Here's how the part is built. I have some questions about the finished solid (model axes, mm). A direction names the side the tool comes from. Round coordinates to 2 decimals unless told otherwise and drop trailing zeros. Write each loop counter-clockwise with the first axis right and the second up, starting at its lowest first coordinate (ties: lowest second). Pieces come first, ordered by that corner, then holes. Notation, with made-up numbers: (48, -26.5) -> (67, -26.5) arc R20 ccw to (67, 2.5) -> close; hole circle Ø8 at (-31.5, 32.5). An arc over 180 degrees is marked (long way). Answer as CSV lines item,"result".
```python
from build123d import *

# Parameters (mm, degrees)
EXTRUDE_1_DEPTH   = 10
SKETCH_2_R        = 19
EXTRUDE_2_DEPTH   = 76
EXTRUDE_3_DEPTH   = 10
SKETCH_4_W        = 35
SKETCH_4_H        = 60
EXTRUDE_4_DEPTH   = 25
SKETCH_5_R        = 30
EXTRUDE_9_DEPTH   = 10
SKETCH_6_R        = 15
EXTRUDE_10_DEPTH  = 10
FILLET_1_R        = 5
SKETCH_7_R        = 7.5
EXTRUDE_11_DEPTH  = 8
SKETCH_8_W        = 30
SKETCH_8_H        = 30
EXTRUDE_12_DEPTH  = 37
FILLET_4_R        = 2
SKETCH_9_W        = 20
SKETCH_9_H        = 17.308382811
EXTRUDE_1_2_DEPTH = 20


with BuildPart() as part:
    # Sketch 1 → Extrude 1 (new body)
    with BuildSketch(Plane.XY):
        Polygon((-25.980762114, 0), (-12.990381057, -22.5), (12.990381057, -22.5), (25.980762114, 0), (12.990381057, 22.5), (-12.990381057, 22.5), align=None)
    extrude(amount=EXTRUDE_1_DEPTH)

    # Sketch 2 → Extrude 2 (add)
    with BuildSketch(Plane(origin=(0, 0, 0), x_dir=(-1, 0, 0), z_dir=(0, 0, -1))):
        with Locations(Location((0, 0, 0), (0, 0, 180))):
            Circle(SKETCH_2_R)
    extrude(amount=EXTRUDE_2_DEPTH)

    # Sketch 3 → Extrude 3 (add)
    with BuildSketch(Plane(origin=(0, 0, -76), x_dir=(-1, 0, 0), z_dir=(0, 0, -1))):
        Polygon((25.980762114, 0), (12.990381057, 22.5), (-12.990381057, 22.5), (-25.980762114, 0), (-12.990381057, -22.5), (12.990381057, -22.5), align=None)
    extrude(amount=EXTRUDE_3_DEPTH)

    # Sketch 4 → Extrude 4 (add)
    with BuildSketch(Plane(origin=(0, 0, 0), x_dir=(1, 0, 0), z_dir=(0, 1, 0))):
        with Locations((0, 38)):
            Rectangle(SKETCH_4_W, SKETCH_4_H)
    extrude(amount=EXTRUDE_4_DEPTH)

    # Sketch 5 → Extrude 9 (add)
    with BuildSketch(Plane(origin=(0, 25, 0), x_dir=(1, 0, 0), z_dir=(0, 1, 0))):
        with Locations(Location((0, 38, 0), (0, 0, 270))):
            Circle(SKETCH_5_R)
    extrude(amount=EXTRUDE_9_DEPTH)

    # Sketch 6 → Extrude 10 (add)
    with BuildSketch(Plane(origin=(0, 35, 0), x_dir=(1, 0, 0), z_dir=(0, 1, 0))):
        with Locations(Location((0, 38, 0), (0, 0, 270))):
            Circle(SKETCH_6_R)
    extrude(amount=EXTRUDE_10_DEPTH)

    # Fillet 1
    fillet_1_edges = [part.edges().sort_by_distance(p)[0] for p in [
        (0, 45, -53),
    ]]
    fillet(fillet_1_edges, radius=FILLET_1_R)

    # Sketch 7 → Extrude 11 (add)
    with BuildSketch(Plane(origin=(0, 45, 0), x_dir=(1, 0, 0), z_dir=(0, 1, 0))):
        with Locations(Location((0, 38, 0), (0, 0, 270))):
            Circle(SKETCH_7_R)
    extrude(amount=EXTRUDE_11_DEPTH)

    # Sketch 8 → Extrude 12 (add)
    with BuildSketch(Plane(origin=(0, 53, 0), x_dir=(1, 0, 0), z_dir=(0, 1, 0))):
        with Locations((0, 38)):
            Rectangle(SKETCH_8_W, SKETCH_8_H)
    extrude(amount=EXTRUDE_12_DEPTH)

    # Fillet 4
    fillet_4_edges = [part.edges().sort_by_distance(p)[0] for p in [
        (0, 35, -68),
    ]]
    fillet(fillet_4_edges, radius=FILLET_4_R)

    # Sketch 9 → Extrude 1 2 (add)
    with BuildSketch(Plane(origin=(0, 0, -53), x_dir=(-1, 0, 0), z_dir=(0, 0, -1))):
        with Locations((0, 79.224035867)):
            Rectangle(SKETCH_9_W, SKETCH_9_H)
    extrude(amount=EXTRUDE_1_2_DEPTH)


solid = part.part
```
1. Suppose I cut it at A-A on z = -38. Please give me the cut outline in (x, y).
Numbers:
outline,"(-30, 25) -> (-17.5, 25) -> (-17.5, 7.4) arc R19 ccw (long way) to (17.5, 7.4) -> (17.5, 25) -> (30, 25) -> (30, 33) arc R2 ccw to (28, 35) -> (15, 35) -> (15, 40) arc R5 ccw to (10, 45) -> (7.5, 45) -> (7.5, 53) -> (15, 53) -> (15, 90) -> (-15, 90) -> (-15, 53) -> (-7.5, 53) -> (-7.5, 45) -> (-10, 45) arc R5 ccw to (-15, 40) -> (-15, 35) -> (-28, 35) arc R2 ccw to (-30, 33) -> close"
2. For pin 1 Ø3 at (x, z) = (0.5, 7) entering from +Y; pin 2 Ø1.7 at (x, z) = (-5, -11) entering from +Y; pin 3 Ø24 at (x, y) = (0.5, 65) entering from -Z, each with a flat end and sliding along its axis, tell me the tip position at first contact or that it passes through.
Numbers:
pin 1,"stops at y = 22.5"
pin 2,"stops at y = 35"
pin 3,"stops at z = -73"
3. If I drill on line 1 (Z direction, x = -22, y = 6); line 2 (Y direction, x = 24, z = -48); line 3 (X direction, y = 15.5, z = -48.5), over which ranges is the centre line in solid material (lowest first)?
Numbers:
line 1,"z = -86 to -76, 0 to 10"
line 2,"y = 25 to 35"
line 3,"x = -17.5 to 17.5"
4. On a 3-axis mill with a long thin cutter (end or side, diameter ignored), from which of +Z, -Z, +X, -X, +Y, -Y can I reach the whole of each face in a straight line? I mean faces 4 (the face through (0.33, 48.944, -45.493)), 5 (the face through (13, 25, -10)), 6 (the face through (0, 71, -23)). Say none if no direction works.
Numbers:
face 4,"none"
face 5,"+Z, +X, +Y"
face 6,"+Z, +X, -X, +Y"
5. Suppose I cut it at D-D on z = -4. Please give me the cut outline in (x, y).
Numbers:
outline,"circle Ø38 at (0, 0)"
6. Suppose I cut it at C-C on z = -78. Please give me the cut outline in (x, y).
Numbers:
outline,"(-25.98, 0) -> (-12.99, -22.5) -> (12.99, -22.5) -> (25.98, 0) -> (12.99, 22.5) -> (-12.99, 22.5) -> close"
7. Suppose I cut it at B-B on y = 78. Please give me the cut outline in (x, z).
Numbers:
outline,"(-15, -53) -> (-10, -53) -> (-10, -73) -> (10, -73) -> (10, -53) -> (15, -53) -> (15, -23) -> (-15, -23) -> close"
8. If we mould it in two halves opening along Y, with no side actions, what happens to faces 1 (the face through (-17.5, 16, -38)), 2 (the face through (0, 87.878, -63)), 3 (the face through (-17.2, 8.44, -76))? For each: released by +Y, released by -Y, zero draft, split by the parting line, or undercut.
Numbers:
face 1,"undercut"
face 2,"released by +Y"
face 3,"zero draft"
